```python
from build123d import *

# Parameters (mm, degrees)
F2_SIZE  = 2
F3_R     = 1
F4_R     = 1
F7_DEPTH = 5


with BuildPart() as f1:
    # F0 (on Right) → F1 (revolve)
    with BuildSketch(Plane.YZ):
        Polygon((0, 25), (-40, 25), (-40, 20), (-80, 20), (-80, 0), (80, 0), (80, 20), (40, 20), (40, 25), align=None)
    revolve(axis=Axis((0, 1.564302, 0), (0, 1, 0)))

    # F2
    f2_edges = [f1.edges().sort_by_distance(p)[0] for p in [
        (0, -80, -20),
        (0, 80, -20),
    ]]
    chamfer(f2_edges, length=F2_SIZE)

    # F3
    f3_edges = [f1.edges().sort_by_distance(p)[0] for p in [
        (0, -40, -20),
    ]]
    fillet(f3_edges, radius=F3_R)

    # F4
    f4_edges = [f1.edges().sort_by_distance(p)[0] for p in [
        (0, 40, -20),
    ]]
    fillet(f4_edges, radius=F4_R)

    # F6 (on offset) → F7 (cut)
    with BuildSketch(Plane.XY.offset(25)):
        with BuildLine():
            Line((-6, 15), (-6, 0))
            Line((-6, 0), (-6, -15))
            ThreePointArc((-6, -15), (0, -21), (6, -15))
            Line((6, -15), (6, 0))
            Line((6, 0), (6, 15))
            ThreePointArc((6, 15), (0, 21), (-6, 15))
        make_face()
    extrude(amount=-F7_DEPTH, mode=Mode.SUBTRACT)


solid = f1.part
```
Check sheet for the modelled part. Datum: model origin and axes. Units: mm. A direction names the side the tool comes from. Coordinates: 2 decimals unless noted, no trailing zeros. Order: outer loops, then holes, each group sorted by start corner. A loop starts at its lowest first (then second) coordinate and runs counter-clockwise, first axis right, second up. Notation, with made-up numbers: (46, 71) -> (75, 71) arc R26 ccw to (75, 97) -> close; hole circle Ø3 at (69.5, 86). An arc over 180 degrees is marked (long way). Write item = value, one per line. Start each with the question number.
1) Cross-section at A-A (z = 0). Enter the section's corners in (x, y).
2) Cross-section at D-D (y = -11.5). Enter the section's corners in (x, z), then the cut area to 3 significant figures.
3) Access from +Z, -Z, +X, -X, +Y, -Y to the whole of each face (thin tool, end or side, straight path). Record for faces 4 (the flat face through (-6, 0, 22)), 5 (the cylindrical face through (-19.524, 59.241, -4.336)), 6 (the cylindrical face through (-19.524, -59.759, -4.336)).
4) Mould release check, pull along X, two halves, no side actions. Record for faces 1 (the conical face through (5.444, 79.875, 17.288)), 2 (the cylindrical face through (0, -21, 23)), 3 (the flat face through (0, 80, 0)): +X half, -X half, draft (parallel to the pull), parting line (faces both ways), or undercut.
5) Cross-section at B-B (x = 0). Enter the section's corners in (y, z), then the cut area to 3 significant figures.
6) Cross-section at C-C (y = 65). Enter the section's corners in (x, z), then the cut area to 3 significant figures.
7) Go/stop test with flat-tipped pins: P1, Ø4, axis at y = -56, z = 4.5, coming from the +X side; P2, Ø1.5, axis at x = 8, z = 17.5, coming from the +Y side; P3, Ø1.3, axis at y = -6.5, z = 23, coming from the -X side; P4, Ø6, axis at x = 1.5, y = -20, coming from the -Z side. Record where each tip stops, or that it passes through.
8) Material ranges on L1, parallel to Y at x = -15.5, z = -16.5; L2, parallel to X at y = 33.5, z = -15; L3, parallel to X at y = 13, z = 22, recorded low to high.
Ans:
q1.outline = (-25, -40) -> (-21, -40) arc R1 cw to (-20, -41) -> (-20, -78) -> (-18, -80) -> (18, -80) -> (20, -78) -> (20, -41) arc R1 cw to (21, -40) -> (25, -40) -> (25, 40) -> (21, 40) arc R1 cw to (20, 41) -> (20, 78) -> (18, 80) -> (-18, 80) -> (-20, 78) -> (-20, 41) arc R1 cw to (-21, 40) -> (-25, 40) -> close
q2.outline = (-6, 20) -> (-6, 24.27) arc R25 ccw (long way) to (6, 24.27) -> (6, 20) -> close
q2.area = 1,910 mm²
q3.face_4 = +Z
q3.face_5 = +Y
q3.face_6 = -Y
q4.face_1 = parting line
q4.face_2 = undercut
q4.face_3 = draft
q5.outline = (-80, -18) -> (-78, -20) -> (-41, -20) arc R1 cw to (-40, -21) -> (-40, -25) -> (40, -25) -> (40, -21) arc R1 cw to (41, -20) -> (78, -20) -> (80, -18) -> (80, 18) -> (78, 20) -> (41, 20) arc R1 cw to (40, 21) -> (40, 25) -> (21, 25) -> (21, 20) -> (-21, 20) -> (-21, 25) -> (-40, 25) -> (-40, 21) arc R1 cw to (-41, 20) -> (-78, 20) -> (-80, 18) -> close
q5.area = 6,980 mm²
q6.outline = circle Ø40 at (0, 0)
q6.area = 1,260 mm²
q7.P1 = 19.84
q7.P2 = 79.51
q7.P3 = -11.2
q7.P4 = -25
q8.L1 = -40 to 40
q8.L2 = -20 to 20
q8.L3 = -11.87 to -6, 6 to 11.87
